from build123d import *

# Parameters (mm, degrees)
BOSS_EXTRUDE1_DEPTH = 6.35
FILLET1_R           = 0.762


with BuildPart() as part:
    # Sketch2 → Boss-Extrude1 (new, symmetric)
    with BuildSketch(Plane(origin=(0, 0, 0), x_dir=(0, 0, -1), z_dir=(1, 0, 0))):
        Polygon((-15.875, 1.27), (-6.985, 1.27), (-6.985, 6.35), (6.985, 6.35), (6.985, 1.27), (15.875, 1.27), (15.875, 2.54), (9.525, 2.54), (9.525, 8.89), (-9.525, 8.89), (-9.525, 2.54), (-15.875, 2.54), align=None)
    extrude(amount=BOSS_EXTRUDE1_DEPTH, both=True)

    # Fillet1
    fillet1_edges = [part.edges().sort_by_distance(p)[0] for p in [
        (-6.35, 2.54, 12.7),
        (-6.35, 5.715, 9.525),
        (6.35, 3.81, 6.985),
        (-6.35, 8.89, 0),
        (-6.35, 5.715, -9.525),
        (-6.35, 2.54, -12.7),
        (-6.35, 3.81, -6.985),
        (-6.35, 6.35, 0),
        (-6.35, 3.81, 6.985),
        (6.35, 6.35, 0),
        (0, 2.54, 15.875),
        (0, 2.54, 9.525),
        (0, 8.89, 9.525),
        (6.35, 3.81, -6.985),
        (0, 8.89, -9.525),
        (0, 2.54, -9.525),
        (0, 2.54, -15.875),
        (6.35, 2.54, -12.7),
        (6.35, 5.715, -9.525),
        (6.35, 8.89, 0),
        (6.35, 5.715, 9.525),
        (6.35, 2.54, 12.7),
    ]]
    fillet(fillet1_edges, radius=FILLET1_R)


solid = part.part
CAD build for the part. Positions are in the model's coordinates, mm. A direction names the side the tool comes from. Round coordinates to 2 decimals unless told otherwise and drop trailing zeros. Write each loop counter-clockwise with the first axis right and the second up, starting at its lowest first coordinate (ties: lowest second). Pieces come first, ordered by that corner, then holes.
(1) 3-axis set-ups, long thin cutter, end or side, ignore diameter. For faces 4 (the face through (0, 2.54, -13)), 5 (the face through (0, 8.89, 0)), 6 (the face through (0, 6.35, 0)), 7 (the face through (0, 2.54, 13)): which of +Z, -Z, +X, -X, +Y, -Y reach the whole face in a straight line?
(2) Slice it at B-B, the plane y = 5.25. Write the cut outline in (x, z) (3 decimals), and give its area (3 significant figures).
(3) Drop flat-ended pins along their axis: P1, Ø1.4, axis at x = 2.5, y = 6.5, coming from the -Z side (3 decimals); P2, Ø1.4, axis at x = -1.5, z = 13, coming from the +Y side; P3, Ø4, axis at x = 4, y = 7, coming from the +Z side (3 decimals). Give the stop position or say it passes through.
(4) Slice it at D-D, the plane z = -12. Write the cut outline in (x, y).
(5) Slice it at A-A, the plane z = 0. Write the cut outline in (x, y), and give its area (3 significant figures).
(6) Slice it at C-C, the plane x = 0.5. Write the cut outline in (y, z) (3 decimals).
(7) Mould opens along Z. For faces 1 (the face through (0, 4, -6.985)), 2 (the face through (0, 6, -9.525)), 3 (the face through (-6.35, 7.3, 0.1)) say: pulls with the +Z half, pulls with the -Z half, needs draft (parallel to the pull), parting line crosses it, or undercut.
(8) Probe line 1 along Z through (x, y) = (3, 4.75) (3 decimals); line 2 along Z through (x, y) = (-1.5, 1.75) (3 decimals); line 3 along Y through (x, z) = (1.5, -1.5). List the from-to ranges inside material, lowest first.
From the geometry:
1. face 4: -Z, +X, -X, +Y
1. face 5: +Z, -Z, +X, -X, +Y
1. face 6: +X, -X, -Y
1. face 7: +Z, +X, -X, +Y
2. outline: (-6.35, -8.763) arc R0.762 ccw to (-5.588, -9.525) - (5.588, -9.525) arc R0.762 ccw to (6.35, -8.763) - (6.35, -7.747) arc R0.762 ccw to (5.588, -6.985) - (-5.588, -6.985) arc R0.762 ccw to (-6.35, -7.747) - close; (-6.35, 7.747) arc R0.762 ccw to (-5.588, 6.985) - (5.588, 6.985) arc R0.762 ccw to (6.35, 7.747) - (6.35, 8.763) arc R0.762 ccw to (5.588, 9.525) - (-5.588, 9.525) arc R0.762 ccw to (-6.35, 8.763) - close
2. area: 63.5 mm2
3. P1: stops at z = -9.525
3. P2: stops at y = 2.54
3. P3: stops at z = 9.525
4. outline: (-6.35, 1.27) - (6.35, 1.27) - (6.35, 1.78) arc R0.76 ccw to (5.59, 2.54) - (-5.59, 2.54) arc R0.76 ccw to (-6.35, 1.78) - close
5. outline: (-6.35, 7.11) arc R0.76 ccw to (-5.59, 6.35) - (5.59, 6.35) arc R0.76 ccw to (6.35, 7.11) - (6.35, 8.13) arc R0.76 ccw to (5.59, 8.89) - (-5.59, 8.89) arc R0.76 ccw to (-6.35, 8.13) - close
5. area: 31.8 mm2
6. outline: (1.27, -15.875) - (1.778, -15.875) arc R0.762 ccw to (2.54, -15.113) - (2.54, -10.287) arc R0.762 cw to (3.302, -9.525) - (8.128, -9.525) arc R0.762 ccw to (8.89, -8.763) - (8.89, 8.763) arc R0.762 ccw to (8.128, 9.525) - (3.302, 9.525) arc R0.762 cw to (2.54, 10.287) - (2.54, 15.113) arc R0.762 ccw to (1.778, 15.875) - (1.27, 15.875) - (1.27, 6.985) - (6.35, 6.985) - (6.35, -6.985) - (1.27, -6.985) - close
7. face 1: undercut
7. face 2: pulls with the -Z half
7. face 3: needs draft
8. line 1: z = -9.525 to -6.985, 6.985 to 9.525
8. line 2: z = -15.875 to -6.985, 6.985 to 15.875
8. line 3: y = 6.35 to 8.89
